Drawing for the job (mm, zero at the part's lowest x, y, z). Give positions to 0.01 mm unless a question says otherwise; leave off trailing zeros. Order: outer loops, then holes, each group sorted by start corner. A loop starts at its lowest first (then second) coordinate and runs counter-clockwise, first axis right, second up. Notation, with made-up numbers: M -18,-30 L -7,-30 A21 ccw -7,-25 Z; hole C -38,31 d4. An arc over 180 degrees is marked long. Answer as a JSON object with one key per item and string values.
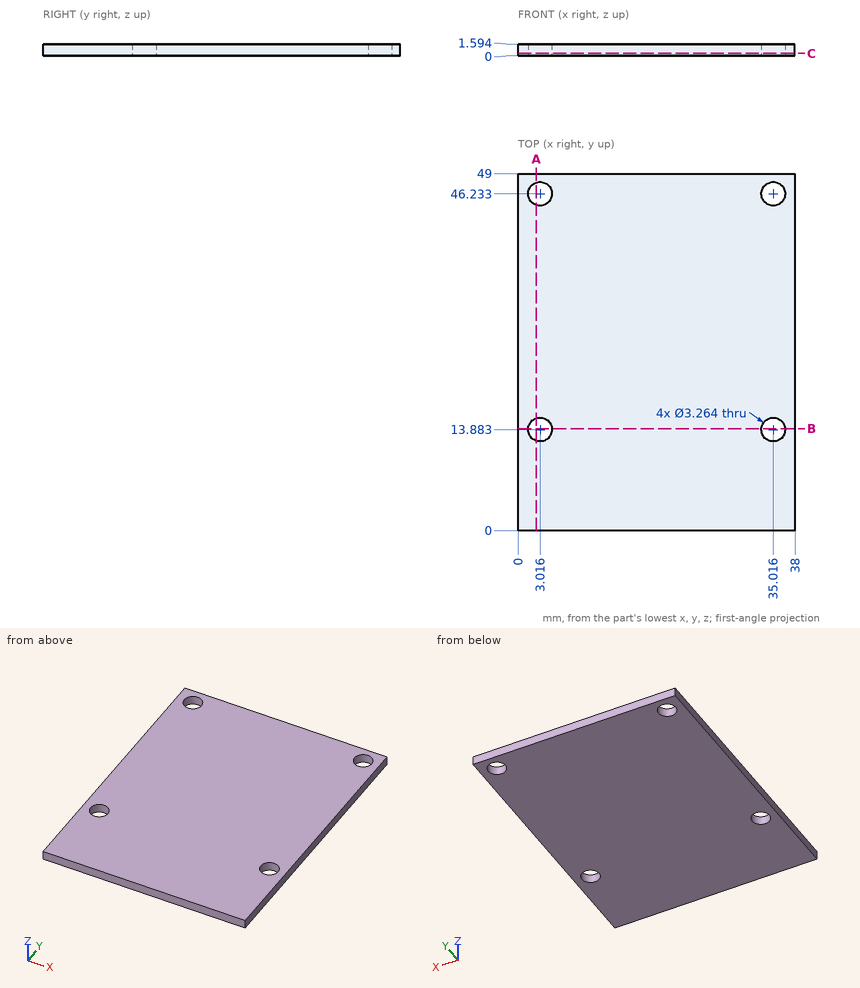
1. Cut at C-C on z = 0.3. Give the cut face in (x, y), plus the area to 3 significant figures.
Worked answers:
{"outline": "M 0,0 L 38,0 L 38,49 L 0,49 Z; hole C 3.02,13.88 d3.26; hole C 3.02,46.23 d3.26; hole C 35.02,13.88 d3.26; hole C 35.02,46.23 d3.26", "area": "1,830 mm^2"}
2. Cut at A-A on x = 2.5. Give the cut face in (y, z) (1 decimal).
Worked answers:
{"outline": "M 0,0 L 12.3,0 L 12.3,1.6 L 0,1.6 Z; M 15.4,0 L 44.7,0 L 44.7,1.6 L 15.4,1.6 Z; M 47.8,0 L 49,0 L 49,1.6 L 47.8,1.6 Z"}
3. Cut at B-B on y = 14. Give the cut face in (x, z).
Worked answers:
{"outline": "M 0,0 L 1.39,0 L 1.39,1.59 L 0,1.59 Z; M 4.64,0 L 33.39,0 L 33.39,1.59 L 4.64,1.59 Z; M 36.64,0 L 38,0 L 38,1.59 L 36.64,1.59 Z"}
4. Probe line 1 along X through (y, z) = (45, 0.95) (1 decimal); line 2 along Y through (x, z) = (3.5, 0.8) (1 decimal); line 3 along X through (y, z) = (46, 1.3). List the from-to ranges inside material, lowest first.
Worked answers:
{"line 1": "x = 0 to 1.9, 4.1 to 33.9, 36.1 to 38", "line 2": "y = 0 to 12.3, 15.4 to 44.7, 47.8 to 49", "line 3": "x = 0 to 1.4, 4.63 to 33.4, 36.63 to 38"}
